```python
from build123d import *

# Parameters (mm, degrees)
SKETCH1_W           = 12.5
SKETCH1_H           = 3.5
BOSS_EXTRUDE1_DEPTH = 0.12


with BuildPart() as part:
    # Sketch1 → Boss-Extrude1 (new body)
    with BuildSketch(Plane.XY.offset(0.12)):
        with Locations((6.25, 1.75)):
            Rectangle(SKETCH1_W, SKETCH1_H)
        with BuildLine():
            ThreePointArc((3.2, 4), (3.053553391, 3.646446609), (2.7, 3.5))
            Line((2.7, 3.5), (9.8, 3.5))
            ThreePointArc((9.8, 3.5), (9.446446609, 3.646446609), (9.3, 4))
            Line((9.3, 4), (3.2, 4))
        make_face()
    extrude(amount=-BOSS_EXTRUDE1_DEPTH)


solid = part.part
```
Can you work these out from the model? Positions are in its coordinate system, mm. Give positions to 0.01 mm unless a question says otherwise; leave off trailing zeros. Loops run counter-clockwise (first coordinate to the right, second up) from the corner with the lowest first, then second, coordinate; pieces in that order, holes last. Notation, with made-up numbers: M -34.75,-21.5 L 20.25,-21.5 A14 ccw 20.25,-13.5 Z; hole C -18,64.25 d4. An arc over 180 degrees is marked long. Use one line per item in the form item = value. Start each with the question number.
(1) I want a section at C-C, the plane x = 1.5. Write out the boundary of the cut face in (y, z), and give its area (3 significant figures).
(2) I want a section at B-B, the plane x = 3. Write out the boundary of the cut face in (y, z), and give its area (3 significant figures).
(3) I want a section at A-A, the plane z = 0.05. Write out the boundary of the cut face in (x, y).
(4) Please list where this line runs through material, in increasing order: line 1 (Y direction, x = 10.25, z = 0.05).
Worked out:
q1.outline = M 0,0 L 3.5,0 L 3.5,0.12 L 0,0.12 Z
q1.area = 0.420 mm²
q2.outline = M 0,0 L 3.6,0 L 3.6,0.12 L 0,0.12 Z
q2.area = 0.432 mm²
q3.outline = M 0,0 L 12.5,0 L 12.5,3.5 L 9.8,3.5 A0.5 cw 9.3,4 L 3.2,4 A0.5 cw 2.7,3.5 L 0,3.5 Z
q4.line_1 = 0 to 3.5
